Input: part model. Units: mm. Frame: model coordinates. Face numbers are marked on the shaded views. Give positions to 0.01 mm unless a question says otherwise; leave off trailing zeros. Loops run counter-clockwise (first coordinate to the right, second up) from the corner with the lowest first, then second, coordinate; pieces in that order, holes last. Notation, with made-up numbers: (-31, 40.25) -> (-2, 40.25) arc R20 ccw to (-2, 74.25) -> close; hole circle Ø3 at (46.25, 52.5). An arc over 180 degrees is marked (long way). One line per question, with ' | ' between items.
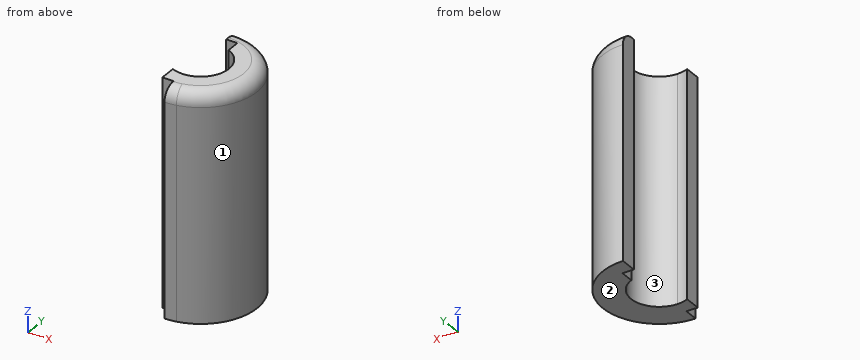
from build123d import *

# Parameters (mm, degrees)
F1_DEPTH = 100
F2_R     = 6


with BuildPart() as f1:
    # F0 (on Top) → F1 (new body)
    with BuildSketch(Plane.XY):
        with BuildLine():
            ThreePointArc((5, 11.456439), (12.236329, -2.553871), (0, -12.5))
            ThreePointArc((0, -12.5), (-2.553871, -12.236329), (-5, -11.456439))
            Line((-5, -11.456439), (-5, -18.75))
            Line((-5, -18.75), (0, -18.75))
            Line((0, -18.75), (0, -25))
            ThreePointArc((0, -25), (2.512724, -24.873404), (5, -24.494897))
            ThreePointArc((5, -24.494897), (24.873404, 2.512724), (0, 25))
            Line((0, 25), (0, 17.5))
            Line((0, 17.5), (5, 17.5))
            Line((5, 17.5), (5, 11.456439))
        make_face()
    extrude(amount=F1_DEPTH)

    # F2
    f2_edges = [f1.edges().sort_by_distance(p)[0] for p in [
        (25, 0, 100),
    ]]
    fillet(f2_edges, radius=F2_R)


solid = f1.part
1. Ray query, line 1 along Y through (x, z) = (1, 8.5); line 2 along Y through (x, z) = (10.5, 49); line 3 along X through (y, z) = (0, 67). Return the intervals inside material, ascending. Write a range as from..to.
Determined:
line 1: y = -24.98..-12.46, 17.5..24.98 | line 2: y = -22.69..-6.78, 6.78..22.69 | line 3: x = 12.5..25
2. Section query A-A (z = 28). Output: boundary loops of the cut face in (x, y).
Determined:
outline: (-5, -18.75) -> (0, -18.75) -> (0, -25) arc R25 ccw to (5, -24.49) arc R25 ccw to (0, 25) -> (0, 17.5) -> (5, 17.5) -> (5, 11.46) arc R12.5 cw to (0, -12.5) arc R12.5 cw to (-5, -11.46) -> close
3. Pull-direction query (Y, two-part tool) for the marked faces 1, 2 and 3; classes: pulls with the +Y half, pulls with the -Y half, needs draft (parallel to the pull), parting line crosses it, or undercut.
Determined:
face 1: parting line crosses it | face 2: needs draft | face 3: undercut
4. Pin query (flat end, axial travel): P1, Ø1.5, axis at y = 17, z = 44.5, coming from the +X side; P2, Ø8.5, axis at y = 22.5, z = 46.5, coming from the -X side; P3, Ø4, axis at x = 2.5, z = 75, coming from the -Y side (3 decimals). Return the tip coordinate at first contact, or that it passes through.
Determined:
P1: stops at x = 19 | P2: stops at x = 0 | P3: stops at y = -24.995
